Autodesk Inventor part; units mm, degrees
ref_plane "YZ Plane" through (0, 0, 0) normal (1, 0, 0) x (0, 1, 0)
ref_plane "XZ Plane" through (0, 0, 0) normal (0, 1, 0) x (-1, 0, 0)
ref_plane "XY Plane" through (0, 0, 0) normal (0, 0, 1) x (1, 0, 0)
sketch "Boceto1" plane through (0, 0, 0) normal (0, 0, 1) x (1, 0, 0)
  line L0 (0, 45) -> (-3.25, 45)
  line L1 (-3.25, 45) -> (-3.25, 65)
  line L2 (-3.25, 65) -> (-0.25, 65)
  line L3 (-0.25, 65) -> (-0.25, 48)
  line L4 (-0.25, 48) -> (3.25, 48)
  line L5 (3.25, 48) -> (3.25, 65)
  line L6 (3.25, 65) -> (6.25, 65)
  line L7 (6.25, 65) -> (6.25, 45)
  line L8 (6.25, 45) -> (3, 45)
  line L9 (3, 0) -> (0, 0)
  line L10 (1.5, 0) -> (1.5, 40) construction
  line L11 (0, 0) -> (0, 15)
  line L12 (0, 15) -> (0, 45)
  line L13 (3, 45) -> (3, 15)
  line L14 (3, 15) -> (3, 0)
  dimension "d1" = 3
  dimension "d4" = 3
  dimension "d5" = 3.5
  dimension "d6" = 9.5
  dimension "d8" = 4.75
  dimension "d9" = 20
  dimension "d20" = 3
  dimension "d27" = 65
extrude "Extrusión1" add sketch "Boceto1" along normal blind 10
sketch "Boceto2" plane through (6.25, 45, 0) normal (1, 0, 0) x (0, 0, -1)
  line L0 (0, 3) -> (-10, 3) construction
  line L1 (0, 0) -> (0, 20) construction
  line L2 (0, 20) -> (-10, 20) construction
  line L3 (-10, 0) -> (-10, 20) construction
  line L4 (0, 0) -> (-10, 0) construction
  line L5 (-10, 0) -> (-10, 20) construction
  line L6 (-10, 20) -> (-10, 3) construction
  line L7 (-10, 14) -> (0, 14) construction
  circle A0 centre (-5, 14) radius 2
  point P0 (0, -45)
  dimension "d15" = 4
  dimension "d16" = 6
extrude "Extrusión2" cut sketch "Boceto2" against normal through all
fillet "Empalme1" radius 3 10 edges at (-1.75, 65, 10) (-1.75, 65, 0) (4.75, 65, 0) (4.75, 65, 10) (0, 45, 5) (3, 45, 5) (6.25, 45, 5) (-3.25, 45, 5) (1.5, 0, 10) (1.5, 0, 0)
sketch "Boceto4" plane through (3, 3, 0) normal (1, 0, 0) x (0, 0, -1)
  arc A0 (-10, 0) -> (-7, -3) centre (-7, 0) ccw construction
  line L0 (0, 0) -> (0, 39) construction
  line L1 (-10, 39) -> (0, 39) construction
  line L2 (-10, 0) -> (-10, 39) construction
  line L3 (-3, -3) -> (-7, -3)
  line L4 (-3, -3) -> (-7, -3) construction
  line L5 (-5, -3) -> (-5, 39) construction
  line L6 (0, 39) -> (-10, 39) construction
  circle A1 centre (-5, 3) radius 2
  arc A2 (-3, -3) -> (0, 0) centre (-3, 0) ccw
  point P0 (0, -3)
  dimension "d28" = 4
  dimension "d29" = 6
extrude "Extrusión3" cut sketch "Boceto4" against normal blind 10
equation "\"d8\" = 0.5 * d6"
properties part number "brazo_servo"
Part model, mm, in its own coordinate system. A direction names the side the tool comes from. Coordinates: 2 decimals unless noted, no trailing zeros. Write each loop counter-clockwise with the first axis right and the second up, starting at its lowest first coordinate (ties: lowest second). Pieces come first, ordered by that corner, then holes.
Item 1: Slice it at C-C (z = 5). Count the separate pieces of the cut face and the enclosed holes in it, and give its area (3 significant figures).
Item 2: Probe line 1 (X direction, y = 59, z = 7.75); line 2 (Y direction, x = 4.65, z = 5); line 3 (Y direction, x = 0.9, z = 5). List the from-to ranges inside material, lowest first.
Item 3: Mould opens along X. For faces 6 (the face through (1, 48, 5)), 7 (the face through (-0.4, 43.5, 5.1)), 8 (the face through (5, 61, 5)) say: released by +X, released by -X, zero draft, split by the parting line, or undercut.
Item 4: Slice it at B-B (y = 59). Write the cut outline in (x, z).
Item 5: Slice it at A-A (y = 6). Write the cut outline in (x, z), and give its area (3 significant figures).
Item 6: Which spindle directions (+Z, -Z, +X, -X, +Y, -Y) get a long thin tool onto all of the face, cutting with end or side? Do faces 1 (the face through (-0.25, 56.6, 4.9)), 2 (the face through (4.77, 64.1, 0.86)), 3 (the face through (0, 21, 5)), 4 (the face through (4.77, 64.14, 9.1)), 5 (the face through (3, 21, 5)). Say none if no direction does.
Item 7: Pin check, flat tips, straight feed: pin 1 (5 mm diameter, centred on y = 24.5, z = 6.5, fed in from -X); pin 2 (3.5 mm diameter, centred on y = 59, z = 5, fed in from +X); pin 3 (3 mm diameter, centred on x = -0.5, z = 9, fed in from +Y). Stop position of each tip, or through.
Item 8: Slice it at D-D (x = -1). Write the cut outline in (y, z).
Results found:
1. separate pieces: 4
1. enclosed holes: 0
1. area: 232 mm2
2. line 1: x = -3.25 to -0.25, 3.25 to 6.25
2. line 2: y = 44.68 to 57, 61 to 65
2. line 3: y = 0 to 4, 8 to 48
3. face 6: undercut
3. face 7: released by -X
3. face 8: zero draft
4. outline: (-3.25, 0) - (-0.25, 0) - (-0.25, 3) - (-3.25, 3) - close; (-3.25, 7) - (-0.25, 7) - (-0.25, 10) - (-3.25, 10) - close; (3.25, 0) - (6.25, 0) - (6.25, 3) - (3.25, 3) - close; (3.25, 7) - (6.25, 7) - (6.25, 10) - (3.25, 10) - close
5. outline: (0, 0) - (3, 0) - (3, 3) - (0, 3) - close; (0, 7) - (3, 7) - (3, 10) - (0, 10) - close
5. area: 18.0 mm2
6. face 1: +Z, -Z, +Y
6. face 2: -Z, +X, -X, +Y
6. face 3: +Z, -Z, -X, -Y
6. face 4: +Z, +X, -X, +Y
6. face 5: +Z, -Z, +X, -Y
7. pin 1: stops at x = 0
7. pin 2: passes through
7. pin 3: stops at y = 64.96
8. outline: (44.24, 0) - (62, 0) arc R3 ccw to (65, 3) - (65, 7) arc R3 ccw to (62, 10) - (44.24, 10) - close; hole circle Ø4 at (59, 5)
